Geometry check sheet. Reference: the model listing, model coordinates, mm. A direction names the side the tool comes from. Round coordinates to 2 decimals unless told otherwise and drop trailing zeros. Write each loop counter-clockwise with the first axis right and the second up, starting at its lowest first coordinate (ties: lowest second). Pieces come first, ordered by that corner, then holes.
Item 1: Cross-section at B-B (z = 2.45). State how many separate pieces and enclosed holes the cut face has, then the cut area to 3 significant figures.
Item 2: Scan lines: probe 1 along Y at (x, z) = (95, 0.6); probe 2 along Y at (x, z) = (81.25, 0.65); probe 3 along X at (y, z) = (27.5, 1.65). Record each from-to range of solid material in increasing order.
Item 3: Access from +Z, -Z, +X, -X, +Y, -Y to the whole of each face (thin tool, end or side, straight path). Record for faces 1 (the face through (64.64, 22.79, 1.48)), 2 (the face through (93.4, 34.57, 1.48)).
Item 4: Depth check by flat-ended pin: P1, Ø8, axis at x = 95, y = 16.25, coming from the -Z side; P2, Ø0.9, axis at x = 54.5, z = 2, coming from the -Y side; P3, Ø1.5, axis at x = 29, z = 2.5, coming from the -Y side. Enter the tip coordinate at first touch or a pass-through.
Item 5: Cross-section at D-D (x = 45). Enter the section's corners in (y, z), then the cut area to 3 significant figures.
Item 6: Cross-section at C-C (y = 16.25). Enter the section's corners in (x, z).
Item 7: Draft check along X on faces 3 (the face through (30.315, 22.762, 1.479)), 4 (the face through (101.645, 80.213, 1.479)), 5 (the face through (-7.5, 47, 1)), 6 (the face through (-0.59, 20.71, 1.52)). Enter one of: pulls with the +X half, pulls with the -X half, needs draft (parallel to the pull), parting line crosses it, or undercut.
Item 8: Cross-section at A-A (x = 95). Enter the section's corners in (y, z), then the cut area to 3 significant figures.
from build123d import *

# Parameters (mm, degrees)
SKETCH_1_R         = 1.6
SKETCH_1_R_2       = 0.95
EXTRUDE_1_DEPTH    = 3
SKETCH1_R          = 4.5
CUT_EXTRUDE1_DEPTH = 25


with BuildPart() as part:
    # 草图1 → 凸台-拉伸1 (new body)
    with BuildSketch(Plane.XY):
        with BuildLine():
            Line((32, 23.279914581), (63, 23.279914581))
            ThreePointArc((63, 23.279914581), (64.664100589, 22.776065464), (65.769230769, 21.433760735))
            Line((65.769230769, 21.433760735), (66.730769231, 19.126068427))
            Line((66.730769231, 19.126068427), (69.29930559, 12.961581165))
            ThreePointArc((69.29930559, 12.961581165), (70.404435771, 11.619276436), (72.068536359, 11.115427319))
            Line((72.068536359, 11.115427319), (99.5, 11.115427319))
            ThreePointArc((99.5, 11.115427319), (101.621320344, 11.994106975), (102.5, 14.115427319))
            Line((102.5, 14.115427319), (102.5, 78.115427319))
            ThreePointArc((102.5, 78.115427319), (101.621320344, 80.236747662), (99.5, 81.115427319))
            Line((99.5, 81.115427319), (-4.5, 81.115427319))
            ThreePointArc((-4.5, 81.115427319), (-6.621320344, 80.236747662), (-7.5, 78.115427319))
            Line((-7.5, 78.115427319), (-7.5, 14.115427319))
            ThreePointArc((-7.5, 14.115427319), (-6.621320344, 11.994106975), (-4.5, 11.115427319))
            Line((-4.5, 11.115427319), (22.931463641, 11.115427319))
            ThreePointArc((22.931463641, 11.115427319), (24.595564229, 11.619276436), (25.70069441, 12.961581165))
            Line((25.70069441, 12.961581165), (28.269230769, 19.126068427))
            Line((28.269230769, 19.126068427), (29.230769231, 21.433760735))
            ThreePointArc((29.230769231, 21.433760735), (30.335899411, 22.776065464), (32, 23.279914581))
        make_face()
        with Locations((0, 34.5)):
            Circle(SKETCH_1_R, mode=Mode.SUBTRACT)
        with Locations((0, 27)):
            Circle(SKETCH_1_R, mode=Mode.SUBTRACT)
        with Locations((95, 34.5)):
            Circle(SKETCH_1_R, mode=Mode.SUBTRACT)
        with Locations((95, 27.1)):
            Circle(SKETCH_1_R, mode=Mode.SUBTRACT)
        with Locations((13.75, 76.079914581)):
            Circle(SKETCH_1_R_2, mode=Mode.SUBTRACT)
        with Locations((81.25, 76.079914581)):
            Circle(SKETCH_1_R_2, mode=Mode.SUBTRACT)
        with Locations((69.5, 20.079914581)):
            Circle(SKETCH_1_R_2, mode=Mode.SUBTRACT)
        with Locations((25.5, 20.079914581)):
            Circle(SKETCH_1_R_2, mode=Mode.SUBTRACT)
    extrude(amount=EXTRUDE_1_DEPTH)

    # Sketch1 → Cut-Extrude1 (cut)
    with BuildSketch(Plane.XY.offset(3)):
        with Locations((0, 16.25)):
            Circle(SKETCH1_R)
        with Locations((95, 16.25)):
            Circle(SKETCH1_R)
    extrude(amount=-CUT_EXTRUDE1_DEPTH, mode=Mode.SUBTRACT)


solid = part.part
Resolved:
1. separate pieces: 1
1. enclosed holes: 10
1. area: 7,030 mm2
2. probe 1: y = 11.12 to 11.75, 20.75 to 25.5, 28.7 to 32.9, 36.1 to 81.12
2. probe 2: y = 11.12 to 75.13, 77.03 to 81.12
2. probe 3: x = -7.5 to -1.52, 1.52 to 93.45, 96.55 to 102.5
3. face 1: +Z, -Z, -Y
3. face 2: +Z, -Z
4. P1: passes through
4. P2: stops at y = 23.28
4. P3: stops at y = 19.08
5. outline: (23.28, 0) - (81.12, 0) - (81.12, 3) - (23.28, 3) - close
5. area: 174 mm2
6. outline: (-7.5, 0) - (-4.5, 0) - (-4.5, 3) - (-7.5, 3) - close; (4.5, 0) - (27.07, 0) - (27.07, 3) - (4.5, 3) - close; (67.93, 0) - (90.5, 0) - (90.5, 3) - (67.93, 3) - close; (99.5, 0) - (102.5, 0) - (102.5, 3) - (99.5, 3) - close
7. face 3: undercut
7. face 4: pulls with the +X half
7. face 5: pulls with the -X half
7. face 6: undercut
8. outline: (11.12, 0) - (11.75, 0) - (11.75, 3) - (11.12, 3) - close; (20.75, 0) - (25.5, 0) - (25.5, 3) - (20.75, 3) - close; (28.7, 0) - (32.9, 0) - (32.9, 3) - (28.7, 3) - close; (36.1, 0) - (81.12, 0) - (81.12, 3) - (36.1, 3) - close
8. area: 164 mm2
